Part model, mm, in its own coordinate system. A direction names the side the tool comes from. Coordinates: 2 decimals unless noted, no trailing zeros. Order: outer loops, then holes, each group sorted by start corner. A loop starts at its lowest first (then second) coordinate and runs counter-clockwise, first axis right, second up.
from build123d import *

# Parameters (mm, degrees)
BOSS_EXTRUDE1_DEPTH = 3.175


with BuildPart() as part:
    # Sketch1 → Boss-Extrude1 (new body)
    with BuildSketch(Plane.XY):
        with BuildLine():
            Line((0, 0), (14.2875, 0))
            ThreePointArc((14.2875, 0), (22.225, 7.9375), (14.2875, 15.875))
            Line((14.2875, 15.875), (0, 15.875))
            Line((0, 15.875), (0, 11.1125))
            Line((0, 11.1125), (6.35, 11.1125))
            Line((6.35, 11.1125), (6.35, 4.7625))
            Line((6.35, 4.7625), (0, 4.7625))
            Line((0, 4.7625), (0, 0))
        make_face()
    extrude(amount=BOSS_EXTRUDE1_DEPTH)


solid = part.part
Q1. Pin check, flat tip, straight feed: pin 1 Ø1 at (y, z) = (4.5, 1.5) entering from +X. Stop position of the tip, or through.
Results list:
pin 1: stops at x = 21.66
Q2. Wall check: line 1 along Y through (x, z) = (1, 1.85) (1 decimal); line 2 along X through (y, z) = (5.5, 0.65); line 3 along X through (y, z) = (14.75, 2.7). Give the ranges that are in metal, low to high.
Results list:
line 1: y = 0 to 4.8, 11.1 to 15.9
line 2: x = 6.35 to 21.84
line 3: x = 0 to 18.36
Q3. Cut at A-A on x = 5.75. Write the cut outline in (y, z) (1 decimal), and give its area (3 significant figures).
Results list:
outline: (0, 0) - (4.8, 0) - (4.8, 3.2) - (0, 3.2) - close; (11.1, 0) - (15.9, 0) - (15.9, 3.2) - (11.1, 3.2) - close
area: 30.2 mm2
Q4. Cut at D-D on x = 20.25. Write the cut outline in (y, z) (3 decimals), and give its area (3 significant figures).
Results list:
outline: (2.698, 0) - (13.177, 0) - (13.177, 3.175) - (2.698, 3.175) - close
area: 33.3 mm2
Q5. Mould opens along Y. For faces 1 (the face through (11, 8, 3.175)), 2 (the face through (3, 4.762, 2)), 3 (the face through (7, 15.875, 2)), 4 (the face through (3, 11.112, 2)) say: pulls with the +Y half, pulls with the -Y half, needs draft (parallel to the pull), parting line crosses it, or undercut.
Results list:
face 1: needs draft
face 2: undercut
face 3: pulls with the +Y half
face 4: undercut
Q6. Cut at C-C on y = 5.75. Write the cut outline in (x, z) (3 decimals), and give its area (3 significant figures).
Results list:
outline: (6.35, 0) - (21.918, 0) - (21.918, 3.175) - (6.35, 3.175) - close
area: 49.4 mm2
Q7. Which spindle directions (+Z, -Z, +X, -X, +Y, -Y) get a long thin tool onto all of the face, cutting with end or side? Do faces 5 (the face through (6.35, 8, 2)), 6 (the face through (22.223, 7.763, 1.565)). Say none if no direction does.
Results list:
face 5: +Z, -Z, -X
face 6: +Z, -Z, +X
